Check sheet for the modelled part. Datum: model origin and axes. Units: mm. Coordinates: 2 decimals unless noted, no trailing zeros. Order: outer loops, then holes, each group sorted by start corner. A loop starts at its lowest first (then second) coordinate and runs counter-clockwise, first axis right, second up.
from build123d import *

# Parameters (mm, degrees)
SKETCH1_R           = 22.225
SKETCH1_R_2         = 2.159
BOSS_EXTRUDE1_DEPTH = 6.35
CUT_EXTRUDE1_DEPTH  = 33.065928179
CIRPATTERN1_COUNT   = 20
BOSS_EXTRUDE2_START = -6.35
SKETCH3_R           = 2.159
BOSS_EXTRUDE2_DEPTH = 6.35


with BuildPart() as part:
    # Sketch1 → Boss-Extrude1 (new body)
    with BuildSketch(Plane(origin=(0, 0, 0), x_dir=(1, 0, 0), z_dir=(0, 1, 0))):
        with Locations(Location((0, 0, 0), (0, 0, 270))):
            Circle(SKETCH1_R)
        with Locations(Location((0, 0, 0), (0, 0, 270))):
            Circle(SKETCH1_R_2, mode=Mode.SUBTRACT)
    extrude(amount=BOSS_EXTRUDE1_DEPTH)

    # Sketch2 → Cut-Extrude1 (cut, through all)
    with BuildSketch(Plane(origin=(0, 6.35, 0), x_dir=(1, 0, 0), z_dir=(0, 1, 0))):
        with BuildLine():
            ThreePointArc((0.664641226, 15.861080576), (0, 15.875), (-0.664641226, 15.861080576))
            ThreePointArc((-0.664641226, 15.861080576), (-1.329908729, 19.128362584), (-2.983334333, 22.023858455))
            ThreePointArc((-2.983334333, 22.023858455), (0, 22.225), (2.983334333, 22.023858455))
            ThreePointArc((2.983334333, 22.023858455), (1.329908729, 19.128362584), (0.664641226, 15.861080576))
        make_face()
    cut_extrude1 = extrude(amount=-CUT_EXTRUDE1_DEPTH, mode=Mode.SUBTRACT)

    # CirPattern1: Cut-Extrude1 ×20 about axis
    cirpattern1_axis = Axis((0, 0, 0), (0, 1, 0))
    for i in range(1, CIRPATTERN1_COUNT):
        add(cut_extrude1.rotate(cirpattern1_axis, i * 360 / CIRPATTERN1_COUNT), mode=Mode.SUBTRACT)

    # Sketch3 → Boss-Extrude2 (add)
    with BuildSketch(Plane(origin=(0, 6.35, 0), x_dir=(1, 0, 0), z_dir=(0, 1, 0)).offset(BOSS_EXTRUDE2_START)):
        with BuildLine():
            Line((3.175, -21.997045256), (3.175, -63.5))
            ThreePointArc((3.175, -63.5), (0, -66.675), (-3.175, -63.5))
            Line((-3.175, -63.5), (-3.175, 4.58754015))
            Line((-3.175, 4.58754015), (10.089938857, 19.80262))
            ThreePointArc((10.089938857, 19.80262), (21.926984622, -3.62739168), (3.175, -21.997045256))
        make_face()
        with Locations(Location((0, -63.5, 0), (0, 0, 270))):
            Circle(SKETCH3_R, mode=Mode.SUBTRACT)
        with Locations(Location((0, 0, 0), (0, 0, 270))):
            Circle(SKETCH3_R, mode=Mode.SUBTRACT)
    extrude(amount=BOSS_EXTRUDE2_DEPTH)


solid = part.part
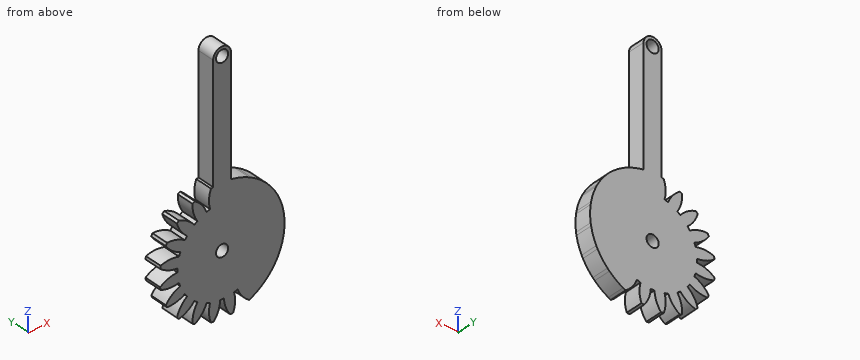
(1) Cross-section at B-B (z = 52). Enter the section's corners in (x, y) (3 decimals).
Filled in:
outline: (-3.175, 0) - (3.175, 0) - (3.175, 6.35) - (-3.175, 6.35) - close
(2) Cross-section at C-C (x = 11.5). Enter the section's corners in (y, z).
Filled in:
outline: (0, -19.02) - (6.35, -19.02) - (6.35, 19.02) - (0, 19.02) - close
(3) Thickness scan on probe 1 along X at (y, z) = (1.75, 0) (3 decimals); probe 2 along X at (y, z) = (1.5, 63.5) (3 decimals); probe 3 along Z at (x, y) = (-0.5, 3.5). Record the ranges inside material, lowest first.
Filled in:
probe 1: x = -15.875 to -2.159, 2.159 to 22.225
probe 2: x = -3.175 to -2.159, 2.159 to 3.175
probe 3: z = -15.87 to -2.1, 2.1 to 61.4, 65.6 to 66.64
(4) Go/stop test with flat-tipped pins: P1, Ø1, axis at x = -6, y = 3, coming from the +Z side; P2, Ø7, axis at x = 0, z = 0, coming from the -Y side; P3, Ø1, axis at y = 4, z = 32.5, coming from the +X side (3 decimals); P4, Ø1.5, axis at x = 9, y = 1, coming from the +Z side. Record where each tip stops, or that it passes through.
Filled in:
P1: stops at z = 16.83
P2: stops at y = 0
P3: stops at x = 3.175
P4: stops at z = 20.64
(5) Cross-section at A-A (y = 3.5). Count the separate pieces of the cut face and the enclosed holes in it, and give its area (3 significant figures).
Filled in:
separate pieces: 1
enclosed holes: 2
area: 1,600 mm2
